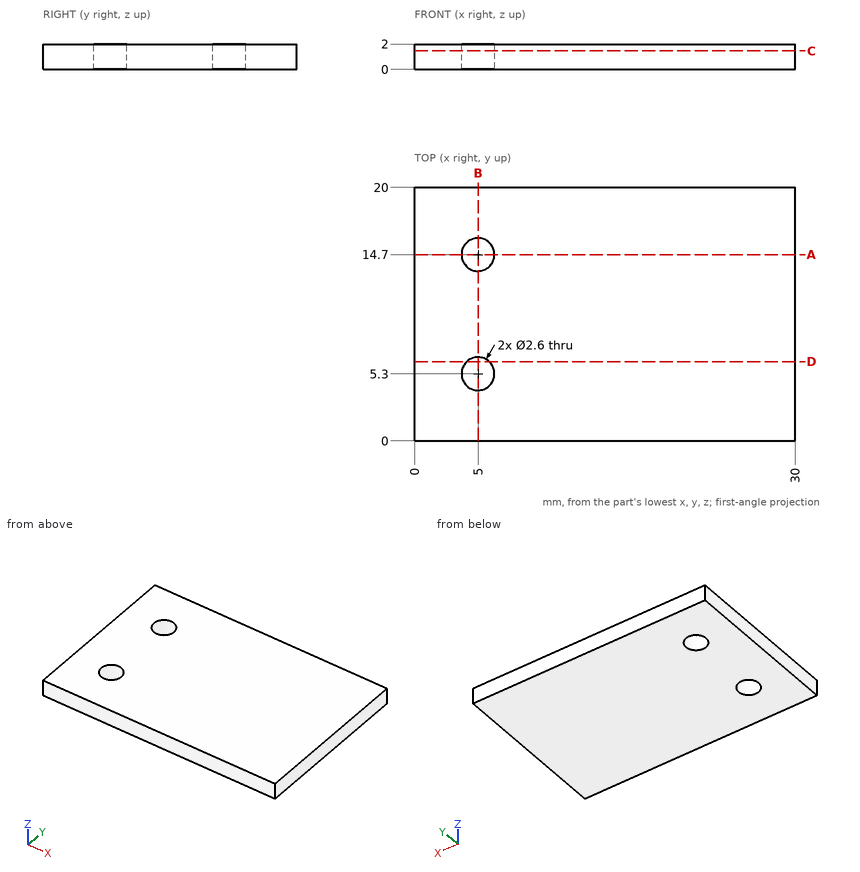
The drawing under review shows one solid part. Ordinate dimensions are in mm from its lowest x, y, z. Round coordinates to 2 decimals unless told otherwise and drop trailing zeros. Write each loop counter-clockwise with the first axis right and the second up, starting at its lowest first coordinate (ties: lowest second). Pieces come first, ordered by that corner, then holes. Notation, with made-up numbers: (81.5, 72.5) -> (132.5, 72.5) arc R24 cw to (132.5, 109.5) -> close; hole circle Ø3 at (33, 37.25). An arc over 180 degrees is marked (long way). One line per question, with ' | ' between items. Start each with the question number.
(1) Insertion check: P1, Ø2.5, axis at x = 5, y = 14.7, coming from the +Z side; P2, Ø1, axis at x = 16.5, y = 3, coming from the -Z side. Each pin has a flat end and moves straight along its axis. Give the tip position at first contact, or say it passes through.
(2) Add section B-B, the plane x = 5. Write out the cut boundary in (y, z).
(3) For line 1 along Y through (x, z) = (5, 1); line 2 along X through (y, z) = (5.75, 1.75), list the stretches that pass through material, from the lowest coordinate up. Write a range as from..to.
(4) Add section A-A, the plane y = 14.7. Write out the cut boundary in (x, z).
(5) Add section D-D, the plane y = 6.25. Write out the cut boundary in (x, z), plus the area to 3 significant figures.
(6) Add section C-C, the plane z = 1.45. Write out the cut boundary in (x, y), plus the area to 3 significant figures.
Answer list:
1) P1: through | P2: z = 0
2) outline: (0, 0) -> (4, 0) -> (4, 2) -> (0, 2) -> close; (6.6, 0) -> (13.4, 0) -> (13.4, 2) -> (6.6, 2) -> close; (16, 0) -> (20, 0) -> (20, 2) -> (16, 2) -> close
3) line 1: 0..4, 6.6..13.4, 16..20 | line 2: 0..3.78, 6.22..30
4) outline: (0, 0) -> (3.7, 0) -> (3.7, 2) -> (0, 2) -> close; (6.3, 0) -> (30, 0) -> (30, 2) -> (6.3, 2) -> close
5) outline: (0, 0) -> (4.11, 0) -> (4.11, 2) -> (0, 2) -> close; (5.89, 0) -> (30, 0) -> (30, 2) -> (5.89, 2) -> close | area: 56.5 mm²
6) outline: (0, 0) -> (30, 0) -> (30, 20) -> (0, 20) -> close; hole circle Ø2.6 at (5, 5.3); hole circle Ø2.6 at (5, 14.7) | area: 589 mm²
